Source: three-view drawing plus pictorial views. Frame: mm from the lowest corner of the part. A direction names the side the tool comes from. Give positions to 0.01 mm unless a question says otherwise; leave off trailing zeros. Order: outer loops, then holes, each group sorted by start corner. A loop starts at its lowest first (then second) coordinate and runs counter-clockwise, first axis right, second up. Notation, with made-up numbers: (-4.75, 20) - (31.25, 20) arc R13 ccw to (31.25, 30) - close; hole circle Ø11 at (-14.75, 0). An arc over 180 degrees is marked (long way). Use one line per item in the form item = value.
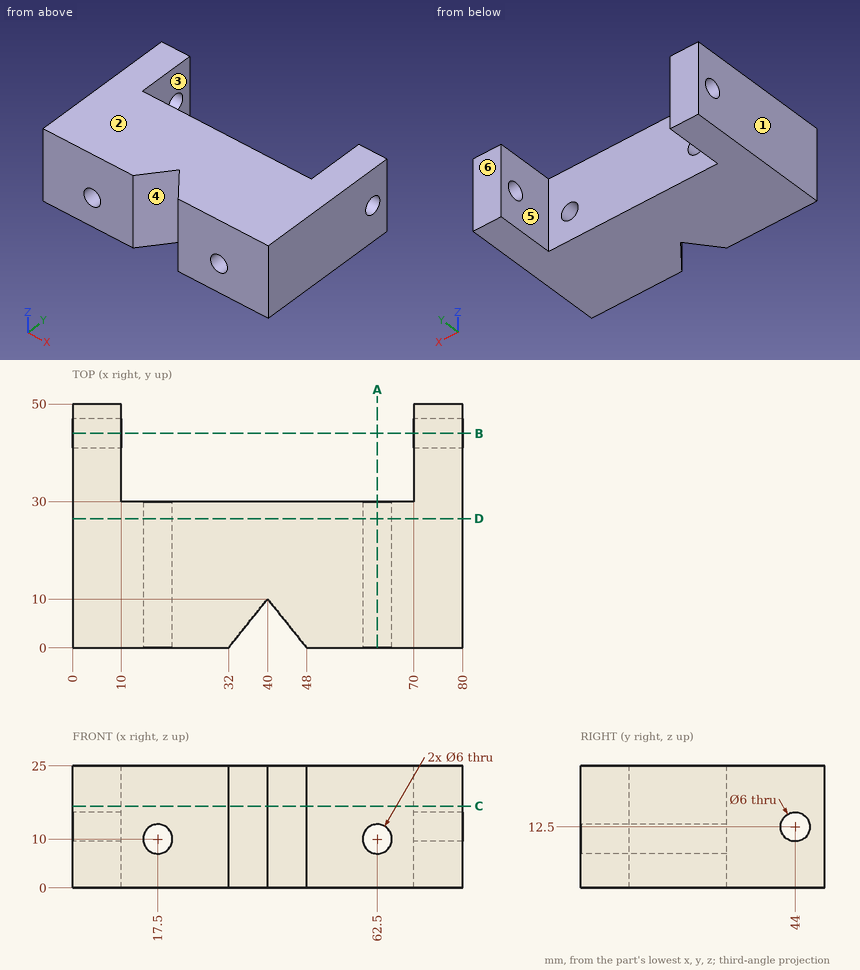
(1) Cut plane A-A on x = 62.5. Output: boundary loops of the cut face in (y, z), plus the area to 3 significant figures.
Computed values:
outline = (0, 0) - (30, 0) - (30, 7) - (0, 7) - close; (0, 13) - (30, 13) - (30, 25) - (0, 25) - close
area = 570 mm²
(2) Cut plane D-D on y = 26.5. Output: boundary loops of the cut face in (x, z).
Computed values:
outline = (0, 0) - (80, 0) - (80, 25) - (0, 25) - close; hole circle Ø6 at (17.5, 10); hole circle Ø6 at (62.5, 10)
(3) Contact query for flat-ended pins moving along their axis: pin 1 Ø5.5 at (x, z) = (62.5, 10) entering from -Y; pin 2 Ø6 at (x, z) = (32.5, 8) entering from +Y; pin 3 Ø4 at (x, z) = (44, 21) entering from -Y. Output: stop coordinate, or through.
Computed values:
pin_1 = through
pin_2 = 30
pin_3 = 2.5
(4) Reachability of the marked faces 4, 5 and 6 from +Z, -Z, +X, -X, +Y, -Y: full face, straight path, thin tool, end or side. Return the list, or none.
Computed values:
face_4 = +Z, -Z, -Y
face_5 = +Z, -Z, +Y
face_6 = +Z, -Z, +X, -X, +Y
(5) Cut plane C-C on z = 16.75. Output: boundary loops of the cut face in (x, y), plus the area to 3 significant figures.
Computed values:
outline = (0, 0) - (32, 0) - (40, 10) - (48, 0) - (80, 0) - (80, 50) - (70, 50) - (70, 30) - (10, 30) - (10, 50) - (0, 50) - close
area = 2,720 mm²
(6) Ray query, line 1 along X through (y, z) = (21.5, 9.75); line 2 along Z through (x, y) = (17.5, 8); line 3 along X through (y, z) = (34, 20). Return the intervals inside material, ascending.
Computed values:
line_1 = 0 to 14.51, 20.49 to 59.51, 65.49 to 80
line_2 = 0 to 7, 13 to 25
line_3 = 0 to 10, 70 to 80
(7) Pull-direction query (X, two-part tool) for the marked faces 1, 2 and 3; classes: released by +X, released by -X, zero draft, split by the parting line, or undercut.
Computed values:
face_1 = released by -X
face_2 = zero draft
face_3 = undercut
(8) Cut plane B-B on y = 44. Output: boundary loops of the cut face in (x, z).
Computed values:
outline = (0, 0) - (10, 0) - (10, 9.5) - (0, 9.5) - close; (0, 15.5) - (10, 15.5) - (10, 25) - (0, 25) - close; (70, 0) - (80, 0) - (80, 9.5) - (70, 9.5) - close; (70, 15.5) - (80, 15.5) - (80, 25) - (70, 25) - close
